```python
from build123d import *

# Parameters (mm, degrees)
F0_W     = 44
F0_H     = 16
F0_R     = 2.5
F1_DEPTH = 12
F2_W     = 13
F2_H     = 13
F2_R     = 2.75
F3_DEPTH = 20


with BuildPart() as f1:
    # F0 (on Top) → F1 (new body)
    with BuildSketch(Plane.XY):
        Rectangle(F0_W, F0_H)
        with Locations((-15, 0)):
            Circle(F0_R, mode=Mode.SUBTRACT)
        with Locations((15, 0)):
            Circle(F0_R, mode=Mode.SUBTRACT)
    extrude(amount=F1_DEPTH)

    # F2 (on face) → F3 (join)
    with BuildSketch(Plane.XY.offset(12)):
        Rectangle(F2_W, F2_H)
        Circle(F2_R, mode=Mode.SUBTRACT)
    extrude(amount=F3_DEPTH)


solid = f1.part
```
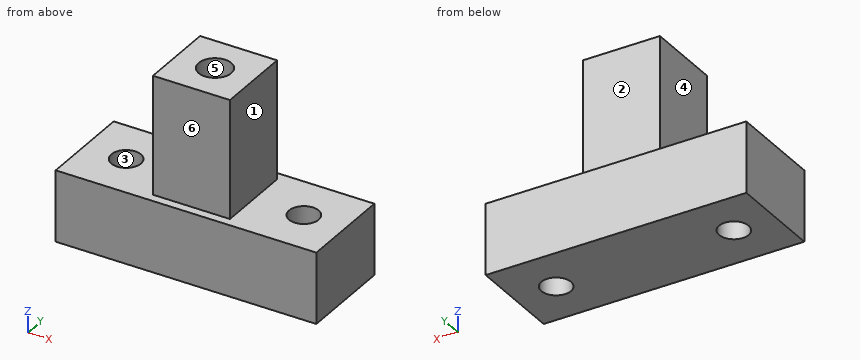
The listing builds one solid part. Answer for the finished solid, in the listing's coordinates (mm). Face numbers are marked on the shaded views. A direction names the side the tool comes from. Round coordinates to 2 decimals unless told otherwise and drop trailing zeros. Loops run counter-clockwise (first coordinate to the right, second up) from the corner with the lowest first, then second, coordinate; pieces in that order, holes last.
1) Consider line 1 (Y direction, x = 0, z = 26); line 2 (X direction, y = 0.75, z = 3); line 3 (Y direction, x = -15, z = 6). Determine where each line is inside the solid, lowest interval first.
Outcome:
line 1: y = -6.5 to -2.75, 2.75 to 6.5
line 2: x = -22 to -17.38, -12.62 to 12.62, 17.38 to 22
line 3: y = -8 to -2.5, 2.5 to 8
2) Given P1, Ø4, axis at y = -3, z = 21, coming from the +X side; P2, Ø3, axis at x = 0, y = -1, coming from the +Z side; P3, Ø6.5, axis at x = 2.5, z = 20, coming from the -Y side, each flat-ended and moving along its own axis, determine where each tip first touches the part or whether it passes through.
Outcome:
P1: stops at x = 6.5
P2: stops at z = 12
P3: stops at y = -6.5
3) A cutting plane is placed at D-D on x = 0. Determine the outline of the cut face in (y, z).
Outcome:
outline: (-8, 0) - (8, 0) - (8, 12) - (6.5, 12) - (6.5, 32) - (2.75, 32) - (2.75, 12) - (-2.75, 12) - (-2.75, 32) - (-6.5, 32) - (-6.5, 12) - (-8, 12) - close
4) For a pull along Y with two mould halves and no side action, classify the marked faces 1, 2 and 3 as released by +Y, released by -Y, zero draft, split by the parting line, or undercut.
Outcome:
face 1: zero draft
face 2: released by +Y
face 3: undercut
5) A cutting plane is placed at B-B on y = 0. Determine the outline of the cut face in (x, z), plus the area to 3 significant figures.
Outcome:
outline: (-22, 0) - (-17.5, 0) - (-17.5, 12) - (-22, 12) - close; (-12.5, 0) - (12.5, 0) - (12.5, 12) - (6.5, 12) - (6.5, 32) - (2.75, 32) - (2.75, 12) - (-2.75, 12) - (-2.75, 32) - (-6.5, 32) - (-6.5, 12) - (-12.5, 12) - close; (17.5, 0) - (22, 0) - (22, 12) - (17.5, 12) - close
area: 558 mm2
6) A cutting plane is placed at A-A on x = -16.5. Determine the outline of the cut face in (y, z).
Outcome:
outline: (-8, 0) - (-2, 0) - (-2, 12) - (-8, 12) - close; (2, 0) - (8, 0) - (8, 12) - (2, 12) - close
7) A cutting plane is placed at C-C on z = 7.5. Determine the outline of the cut face in (x, y), plus the area to 3 significant figures.
Outcome:
outline: (-22, -8) - (22, -8) - (22, 8) - (-22, 8) - close; hole circle Ø5 at (-15, 0); hole circle Ø5 at (15, 0)
area: 665 mm2
8) For the marked faces 4, 5 and 6, determine the directions among +Z, -Z, +X, -X, +Y, -Y from which every point of the face is accessible in a straight line to the end or side of a thin tool.
Outcome:
face 4: +Z, -X, +Y, -Y
face 5: +Z
face 6: +Z, +X, -X, -Y
